The model under review builds one solid part; all positions refer to its coordinate system, in mm. Coordinates: 2 decimals unless noted, no trailing zeros. Order: outer loops, then holes, each group sorted by start corner. A loop starts at its lowest first (then second) coordinate and runs counter-clockwise, first axis right, second up. Notation, with made-up numbers: (-27.5, 71.5) - (21.5, 71.5) arc R13 ccw to (21.5, 93.5) - close; hole circle Ø11 at (65, -2). An arc over 180 degrees is marked (long way). Answer in a Markdown table with one row per item.
```python
from build123d import *

# Parameters (mm, degrees)
ESQUISSE1_W        = 97
ESQUISSE1_H        = 62
BOSS_EXTRU_1_DEPTH = 2
ESQUISSE3_W        = 1.51
ESQUISSE3_H        = 3
BOSS_EXTRU_3_DEPTH = 1.51
ESQUISSE4_W        = 5
ESQUISSE4_H        = 10
BOSS_EXTRU_4_DEPTH = 5


with BuildPart() as part:
    # Esquisse1 → Boss.-Extru.1 (new body)
    with BuildSketch(Plane.XY):
        with Locations((0.382294712, -7.666666667)):
            Rectangle(ESQUISSE1_W, ESQUISSE1_H)
    extrude(amount=BOSS_EXTRU_1_DEPTH)

    # Esquisse3 → Boss.-Extru.3 (add)
    with BuildSketch(Plane.XY.offset(2)):
        with Locations((-47.362705288, -7.666666667)):
            Rectangle(ESQUISSE3_W, ESQUISSE3_H)
    extrude(amount=BOSS_EXTRU_3_DEPTH)

    # Esquisse4 → Boss.-Extru.4 (add)
    with BuildSketch(Plane.XY.offset(3.51)):
        with Locations((-45.617705288, -7.666666667)):
            Rectangle(ESQUISSE4_W, ESQUISSE4_H)
    extrude(amount=BOSS_EXTRU_4_DEPTH)


solid = part.part
```
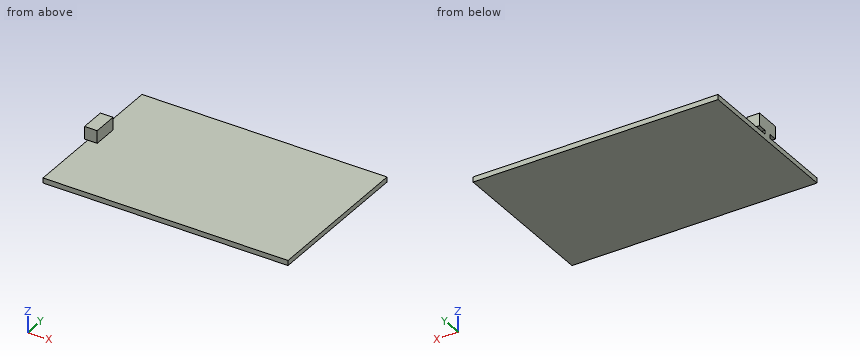
Item 1: Clearance check with flat-ended pins moving along their axes: pin 1 Ø2 at (x, y) = (-3.5, -1.5) entering from +Z; pin 2 Ø1.7 at (y, z) = (-7.5, 3) entering from +X; pin 3 Ø2.5 at (x, y) = (-45, -6) entering from -Z; pin 4 Ø4 at (x, z) = (-46.5, 5) entering from -Y. State where each tip first meets the part, or that it passes through.
Check values:
| item | result |
|---|---|
| pin 1 | z = 2 |
| pin 2 | x = -43.12 |
| pin 3 | z = 0 |
| pin 4 | y = -12.67 |
Item 2: We need section C-C, the plane z = 6.5. Write out the cut boundary in (x, y).
Check values:
| item | result |
|---|---|
| outline | (-48.12, -12.67) - (-43.12, -12.67) - (-43.12, -2.67) - (-48.12, -2.67) - close |
Item 3: We need section A-A, the plane y = -11. Write out the cut boundary in (x, z), then the cut area to 3 significant figures.
Check values:
| item | result |
|---|---|
| outline | (-48.12, 0) - (48.88, 0) - (48.88, 2) - (-48.12, 2) - close; (-48.12, 3.51) - (-43.12, 3.51) - (-43.12, 8.51) - (-48.12, 8.51) - close |
| area | 219 mm^2 |
Item 4: To check wall thickness, follow line 1 (Z direction, x = -29, y = -11); line 2 (X direction, y = -7, z = 4). State the ranges of each line that lie inside material, in increasing order. Write a range as from..to.
Check values:
| item | result |
|---|---|
| line 1 | 0..2 |
| line 2 | -48.12..-43.12 |
Item 5: We need section B-B, the plane x = 21. Write out the cut boundary in (y, z), then the cut area to 3 significant figures.
Check values:
| item | result |
|---|---|
| outline | (-38.67, 0) - (23.33, 0) - (23.33, 2) - (-38.67, 2) - close |
| area | 124 mm^2 |
